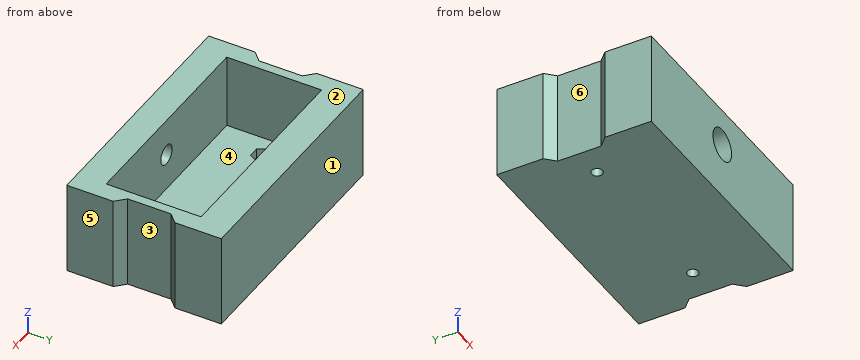
```python
from build123d import *

# Parameters (mm, degrees)
SKETCH1_W               = 80
SKETCH1_H               = 50
BOSS_EXTRUDE1_DEPTH     = 30
CUT_EXTRUDE1_DEPTH      = 56.901699437
CUT_EXTRUDE1_DEPTH_BACK = 56.901699437
SKETCH2_W               = 6
SKETCH2_H               = 20
CHAMFER1_SIZE           = 3
CUT_EXTRUDE2_START      = 30
SKETCH3_W               = 68
SKETCH3_H               = 30
CUT_EXTRUDE2_DEPTH      = 24
SKETCH4_R               = 3.2
CUT_EXTRUDE3_DEPTH      = 56.901699437
CUT_EXTRUDE4_DEPTH      = 56.901699437
CUT_EXTRUDE4_DEPTH_BACK = 56.901699437
SKETCH5_R               = 1.75
CUT_EXTRUDE5_START      = 6
CUT_EXTRUDE5_DEPTH      = 3
CUT_EXTRUDE6_START      = -25
SKETCH7_R               = 5.25
CUT_EXTRUDE6_DEPTH      = 6
CUT_EXTRUDE8_START      = 30
SKETCH10_W              = 68
SKETCH10_H              = 0.7
CUT_EXTRUDE8_DEPTH      = 24


with BuildPart() as part:
    # Sketch1 → Boss-Extrude1 (new body)
    with BuildSketch(Plane.XY):
        Rectangle(SKETCH1_W, SKETCH1_H)
    extrude(amount=BOSS_EXTRUDE1_DEPTH)

    # Sketch2 → Cut-Extrude1 (cut, two sides: drawn at the far end of the back side and taken through both)
    with BuildSketch(Plane.XY.offset(-CUT_EXTRUDE1_DEPTH_BACK)):
        with Locations((-40, 0)):
            Rectangle(SKETCH2_W, SKETCH2_H)
        with Locations((40, 0)):
            Rectangle(SKETCH2_W, SKETCH2_H)
    extrude(amount=CUT_EXTRUDE1_DEPTH + CUT_EXTRUDE1_DEPTH_BACK, mode=Mode.SUBTRACT)

    # Chamfer1
    chamfer1_edges = [part.edges().sort_by_distance(p)[0] for p in [
        (37, 10, 15),
        (37, -10, 15),
        (-37, -10, 15),
        (-37, 10, 15),
    ]]
    chamfer(chamfer1_edges, length=CHAMFER1_SIZE - 0.0001)  # a hair under: the kernel refuses the full size

    # Sketch3 → Cut-Extrude2 (cut)
    with BuildSketch(Plane.XY.offset(CUT_EXTRUDE2_START)):
        Rectangle(SKETCH3_W, SKETCH3_H)
    extrude(amount=-CUT_EXTRUDE2_DEPTH, mode=Mode.SUBTRACT)

    # Sketch4 → Cut-Extrude3 (cut, through all)
    with BuildSketch(Plane(origin=(0, 0, 0), x_dir=(1, 0, 0), z_dir=(0, 1, 0))):
        with Locations(Location((0, -18, 0), (0, 0, 270))):
            Circle(SKETCH4_R)
    extrude(amount=-CUT_EXTRUDE3_DEPTH, mode=Mode.SUBTRACT)

    # Sketch5 → Cut-Extrude4 (cut, two sides: drawn at the far end of the back side and taken through both)
    with BuildSketch(Plane.XY.offset(-CUT_EXTRUDE4_DEPTH_BACK)):
        with Locations(Location((27, 0, 0), (0, 0, 180))):
            Circle(SKETCH5_R)
        with Locations(Location((-27, 0, 0), (0, 0, 180))):
            Circle(SKETCH5_R)
    extrude(amount=CUT_EXTRUDE4_DEPTH + CUT_EXTRUDE4_DEPTH_BACK, mode=Mode.SUBTRACT)

    # Sketch6 → Cut-Extrude5 (cut)
    with BuildSketch(Plane.XY.offset(CUT_EXTRUDE5_START)):
        Polygon((-23.535898385, 0), (-25.267949192, 3), (-28.732050808, 3), (-30.464101615, 0), (-28.732050808, -3), (-25.267949192, -3), align=None)
        Polygon((30.464101615, 0), (28.732050808, 3), (25.267949192, 3), (23.535898385, 0), (25.267949192, -3), (28.732050808, -3), align=None)
    extrude(amount=-CUT_EXTRUDE5_DEPTH, mode=Mode.SUBTRACT)

    # Sketch7 → Cut-Extrude6 (cut)
    with BuildSketch(Plane(origin=(0, 0, 0), x_dir=(1, 0, 0), z_dir=(0, 1, 0)).offset(CUT_EXTRUDE6_START)):
        with Locations(Location((0, -18, 0), (0, 0, 270))):
            Circle(SKETCH7_R)
    extrude(amount=CUT_EXTRUDE6_DEPTH, mode=Mode.SUBTRACT)

    # Sketch10 → Cut-Extrude8 (cut)
    with BuildSketch(Plane.XY.offset(CUT_EXTRUDE8_START)):
        with Locations((0, -15.35)):
            Rectangle(SKETCH10_W, SKETCH10_H)
    extrude(amount=-CUT_EXTRUDE8_DEPTH, mode=Mode.SUBTRACT)


solid = part.part
```
Input: part model. Units: mm. Frame: model coordinates. Face numbers are marked on the shaded views. A direction names the side the tool comes from. Give positions to 0.01 mm unless a question says otherwise; leave off trailing zeros. Order: outer loops, then holes, each group sorted by start corner. A loop starts at its lowest first (then second) coordinate and runs counter-clockwise, first axis right, second up.
1. Set-up query: the marked faces 4, 5 and 6. Return all of +Z, -Z, +X, -X, +Y, -Y with unobstructed straight access to the full face (end or side cutting, diameter ignored); none if empty.
Computed:
face 4: +Z
face 5: +Z, -Z, +X, +Y, -Y
face 6: +Z, -Z, -X
2. Cut plane B-B (x = 0). Return loops of the section in (y, z).
Computed:
outline: (-25, 0) - (25, 0) - (25, 30) - (15, 30) - (15, 6) - (-15.7, 6) - (-15.7, 14.8) - (-19, 14.8) - (-19, 12.75) - (-25, 12.75) - close; (-25, 23.25) - (-19, 23.25) - (-19, 21.2) - (-15.7, 21.2) - (-15.7, 30) - (-25, 30) - close
3. Line query: probe 1 along Y at (x, z) = (-2.5, 28.5); probe 2 along X at (y, z) = (-1.5, 9); probe 3 along X at (y, z) = (-14.5, 24.5). Output: solid intervals per line, ascending.
Computed:
probe 1: y = -25 to -15.7, 15 to 25
probe 2: x = -37 to -34, 34 to 37
probe 3: x = -40 to -34, 34 to 40
4. Draft query along Y for the marked faces 1, 2 and 3. Return one class per face: released by +Y, released by -Y, zero draft, split by the parting line, or undercut.
Computed:
face 1: released by +Y
face 2: zero draft
face 3: undercut
5. Cut plane D-D (x = 33). Return loops of the section in (y, z).
Computed:
outline: (-25, 0) - (25, 0) - (25, 30) - (15, 30) - (15, 6) - (-15.7, 6) - (-15.7, 30) - (-25, 30) - close
6. Pin query (flat end, axial travel): pin 1 Ø1 at (y, z) = (7, 20) entering from +X; pin 2 Ø6.5 at (x, y) = (25.5, 1) entering from +Z; pin 3 Ø12 at (y, z) = (3, 17.5) entering from +X. Return the tip coordinate at first contact, or that it passes through.
Computed:
pin 1: stops at x = 37.5
pin 2: stops at z = 6
pin 3: stops at x = 39
